Geometry check sheet. Reference: drawing and pictorial views, mm from the part's lowest x, y, z. A direction names the side the tool comes from. Round coordinates to 2 decimals unless told otherwise and drop trailing zeros. Order: outer loops, then holes, each group sorted by start corner. A loop starts at its lowest first (then second) coordinate and runs counter-clockwise, first axis right, second up.
(1) Sectioned sample at C-C, the plane y = 11.5. Enter the section's corners in (x, z).
(2) Sectioned sample at A-A, the plane x = 19. Enter the section's corners in (y, z), and give its area (3 significant figures).
(3) Sectioned sample at B-B, the plane z = 22. Enter the section's corners in (x, y).
(4) Tool access check on the marked faces 1 and 2. Record the directions out of +Z, -Z, +X, -X, +Y, -Y that give a thin tool (end or side, any length) a straight path to the whole face; none if there is none.
(5) Thickness scan on probe 1 along Y at (x, z) = (19, 15); probe 2 along X at (y, z) = (12, 9); probe 3 along Z at (x, y) = (22, 3). Record the ranges inside material, lowest first.
(6) Depth check by flat-ended pin: pin 1 (5 mm diameter, centred on x = 12.5, y = 9.5, fed in from -Z). Enter the tip coordinate at first touch or a pass-through.
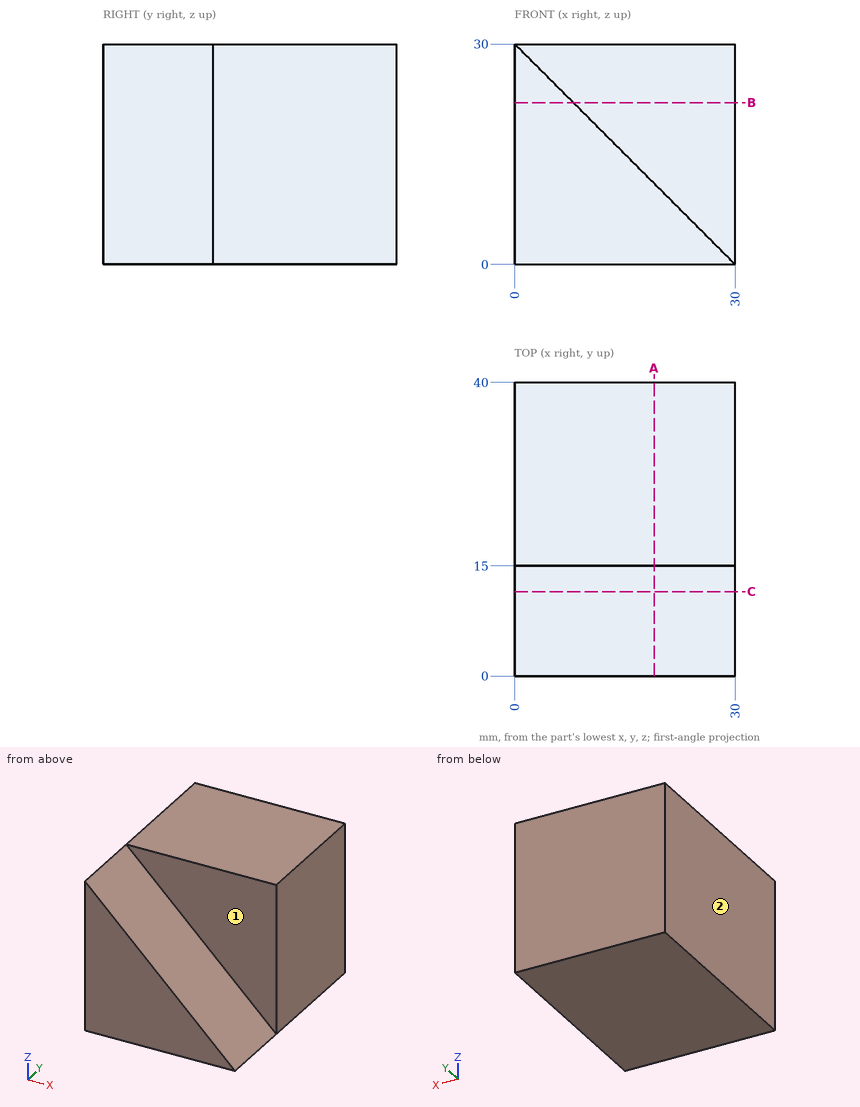
Derived:
1. outline: (0, 0) - (30, 0) - (0, 30) - close
2. outline: (0, 0) - (40, 0) - (40, 30) - (15, 30) - (15, 11) - (0, 11) - close
2. area: 915 mm2
3. outline: (0, 0) - (8, 0) - (8, 15) - (30, 15) - (30, 40) - (0, 40) - close
4. face 1: +Z, +X, -Y
4. face 2: +Z, -Z, -X, +Y, -Y
5. probe 1: y = 15 to 40
5. probe 2: x = 0 to 21
5. probe 3: z = 0 to 8
6. pin 1: stops at z = 0
